Design review of the part built by this model. Coordinates are the model's own, in mm. A direction names the side the tool comes from. Coordinates: 2 decimals unless noted, no trailing zeros. Write each loop counter-clockwise with the first axis right and the second up, starting at its lowest first coordinate (ties: lowest second). Pieces come first, ordered by that corner, then holes.
Q1. Take a section at A-A, the plane y = 0. Write out the cut boundary in (x, z).
Q2. Take a section at C-C, the plane z = 25. Write out the cut boundary in (x, y), plus the area to 3 significant figures.
Q3. Take a section at D-D, the plane x = 39. Write out the cut boundary in (y, z), plus the area to 3 significant figures.
Q4. For pin 1 Ø18 at (x, y) = (0, 0) entering from -Z; pin 2 Ø1.5 at (x, y) = (-11.5, -19) entering from +Z; pin 3 Ø9 at (x, y) = (-23.51, 32.36) entering from +Z; pin 4 Ø2 at (x, z) = (6.5, 4) entering from -Y, all flat-tipped, find the tip position at first contact; note any pin that passes through.
Q5. Take a section at B-B, the plane x = 0. Write out the cut boundary in (y, z).
Q6. The part is to be moulded in two halves that separate along Y. For faces 1 (the cylindrical face through (-29.97, 1.32, 23.83)), 2 (the flat face through (-11, -19, 22)), 3 (the flat face through (10, -10, 0)), say which applies: released by +Y, released by -Y, zero draft, split by the parting line, or undercut.
Q7. For faces 4 (the cylindrical face through (10.46, 16.61, 29.1)), 5 (the cylindrical face through (-35.367, -16.077, 5.916)), list the 3-axis set-ups (+Z, -Z, +X, -X, +Y, -Y) from which the entire face can be reached by the end or side of a thin tool; tool diameter is ignored.
Q8. For L1, parallel to X at y = 40.5, z = 11; L2, parallel to X at y = 19, z = 10; L3, parallel to Y at x = 17.5, z = 3.5, list the stretches that pass through material, from the lowest coordinate up.
from build123d import *

# Parameters (mm, degrees)
SKETCH_1_R          = 47
EXTRUDE_1_DEPTH     = 12
SKETCH_2_R          = 30
EXTRUDE_2_DEPTH     = 36
SKETCH_3_R          = 10
CUT_EXTRUDE_1_DEPTH = 37
SKETCH_4_R          = 2.75
SKETCH_4_R_2        = 2.1
CUT_EXTRUDE_2_DEPTH = 13
SKETCH_5_R          = 2.5
CUT_EXTRUDE_3_DEPTH = 14


with BuildPart() as part:
    # 草图1 → 凸台-拉伸1 (new body)
    with BuildSketch(Plane.XY):
        Circle(SKETCH_1_R)
    extrude(amount=EXTRUDE_1_DEPTH)

    # 草图2 → 凸台-拉伸2 (add)
    with BuildSketch(Plane.XY):
        Circle(SKETCH_2_R)
    extrude(amount=EXTRUDE_2_DEPTH)

    # 草图3 → 切除-拉伸1 (cut)
    with BuildSketch(Plane(origin=(0, 0, 0), x_dir=(-1, 0, 0), z_dir=(0, 0, -1))):
        Circle(SKETCH_3_R)
    extrude(amount=-CUT_EXTRUDE_1_DEPTH, mode=Mode.SUBTRACT)

    # 草图4 → 切除-拉伸2 (cut)
    with BuildSketch(Plane(origin=(0, 0, 0), x_dir=(-1, 0, 0), z_dir=(0, 0, -1))):
        with Locations((-38.042994, -12.358424)):
            Circle(SKETCH_4_R)
        with Locations((-32.362074, -23.509491)):
            Circle(SKETCH_4_R)
        with Locations((-23.513329, -32.359286)):
            Circle(SKETCH_4_R)
        with Locations((-12.362935, -38.041528)):
            Circle(SKETCH_4_R)
        with Locations((12.358424, -38.042994)):
            Circle(SKETCH_4_R)
        with Locations((23.509491, -32.362074)):
            Circle(SKETCH_4_R)
        with Locations((32.359286, -23.513329)):
            Circle(SKETCH_4_R)
        with Locations((38.041528, -12.362935)):
            Circle(SKETCH_4_R)
        with Locations((38.042994, 12.358424)):
            Circle(SKETCH_4_R)
        with Locations((32.362074, 23.509491)):
            Circle(SKETCH_4_R)
        with Locations((23.513329, 32.359286)):
            Circle(SKETCH_4_R)
        with Locations((12.362935, 38.041528)):
            Circle(SKETCH_4_R)
        with Locations((-12.358424, 38.042994)):
            Circle(SKETCH_4_R)
        with Locations((-23.509491, 32.362074)):
            Circle(SKETCH_4_R)
        with Locations((-32.359286, 23.513329)):
            Circle(SKETCH_4_R)
        with Locations((-38.041528, 12.362935)):
            Circle(SKETCH_4_R)
        with Locations((-35.640260968, 18.15961999)):
            Circle(SKETCH_4_R_2)
        with Locations((-18.15961999, 35.640260968)):
            Circle(SKETCH_4_R_2)
        with Locations((18.15961999, 35.640260968)):
            Circle(SKETCH_4_R_2)
        with Locations((35.640260968, 18.15961999)):
            Circle(SKETCH_4_R_2)
        with Locations((35.640260968, -18.15961999)):
            Circle(SKETCH_4_R_2)
        with Locations((18.15961999, -35.640260968)):
            Circle(SKETCH_4_R_2)
        with Locations((-18.15961999, -35.640260968)):
            Circle(SKETCH_4_R_2)
        with Locations((-35.640260968, -18.15961999)):
            Circle(SKETCH_4_R_2)
    extrude(amount=-CUT_EXTRUDE_2_DEPTH, mode=Mode.SUBTRACT)

    # 草图5 → 切除-拉伸3 (cut)
    with BuildSketch(Plane.XY.offset(36)):
        with Locations((22, 0)):
            Circle(SKETCH_5_R)
        with Locations((11, 19.052558883)):
            Circle(SKETCH_5_R)
        with Locations((-11, 19.052558883)):
            Circle(SKETCH_5_R)
        with Locations((-22, 0)):
            Circle(SKETCH_5_R)
        with Locations((-11, -19.052558883)):
            Circle(SKETCH_5_R)
        with Locations((11, -19.052558883)):
            Circle(SKETCH_5_R)
    extrude(amount=-CUT_EXTRUDE_3_DEPTH, mode=Mode.SUBTRACT)


solid = part.part
Responses:
1. outline: (-47, 0) - (-10, 0) - (-10, 36) - (-19.5, 36) - (-19.5, 22) - (-24.5, 22) - (-24.5, 36) - (-30, 36) - (-30, 12) - (-47, 12) - close; (10, 0) - (47, 0) - (47, 12) - (30, 12) - (30, 36) - (24.5, 36) - (24.5, 22) - (19.5, 22) - (19.5, 36) - (10, 36) - close
2. outline: circle Ø60 at (0, 0); hole circle Ø5 at (-22, 0); hole circle Ø5 at (-11, -19.05); hole circle Ø5 at (-11, 19.05); hole circle Ø20 at (0, 0); hole circle Ø5 at (11, -19.05); hole circle Ø5 at (11, 19.05); hole circle Ø5 at (22, 0)
2. area: 2,400 mm2
3. outline: (-26.23, 0) - (-14.94, 0) - (-14.94, 12) - (-26.23, 12) - close; (-9.78, 0) - (9.79, 0) - (9.79, 12) - (-9.78, 12) - close; (14.94, 0) - (26.23, 0) - (26.23, 12) - (14.94, 12) - close
3. area: 506 mm2
4. pin 1: passes through
4. pin 2: stops at z = 22
4. pin 3: stops at z = 12
4. pin 4: stops at y = -46.68
5. outline: (-47, 0) - (-10, 0) - (-10, 36) - (-30, 36) - (-30, 12) - (-47, 12) - close; (10, 0) - (47, 0) - (47, 12) - (30, 12) - (30, 36) - (10, 36) - close
6. face 1: split by the parting line
6. face 2: undercut
6. face 3: zero draft
7. face 4: +Z
7. face 5: +Z, -Z
8. L1: x = -23.85 to -13.6, -11.13 to 11.12, 13.59 to 23.85
8. L2: x = -42.99 to -37.56, -33.72 to 33.72, 37.56 to 42.99
8. L3: y = -43.62 to -37.63, -33.65 to 33.65, 37.63 to 43.62
